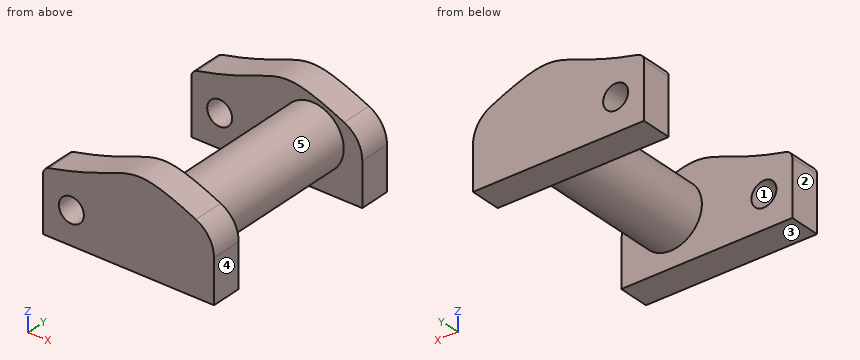
from build123d import *

# Parameters (mm, degrees)
F1_DEPTH = 25.4
F2_R     = 25.4
F3_DEPTH = 127
F6_R     = 25.3967781552
F7_R     = 10.211273354
F8_DEPTH = 211.42987


# Not quite as in the source:
# - a feature of the source that left no trace in its solid (it failed there, or was rolled back) is left out
# - a pattern or mirror of a feature is missing from the dataset's text; its kind, count and spacing are read off the source's solid


with BuildPart() as f1:
    # F0 (on Front) → F1 (new body)
    with BuildSketch(Plane.XZ):
        with BuildLine():
            Line((-140.086213054, 0), (0, 0))
            Line((0, 0), (0, 51.7864115536))
            add(Edge.make_bspline(
                [(-135.121182604, 51.4369904306), (-57.8541277154, 68.705081156), (-79.1493766813, 89.948796737), (0, 51.7864115536)],
                knots=[0.0132853618, 0.0132853618, 0.0132853618, 0.0132853618, 0.6502691411, 0.6502691411, 0.6502691411, 0.6502691411], degree=3))
            ThreePointArc((-135.121182604, 51.4369904306), (-138.6918692488, 49.210252186), (-140.086213054, 45.2398653435))
            Line((-140.086213054, 45.2398653435), (-140.086213054, 0))
        make_face()
    extrude(amount=F1_DEPTH)


with BuildPart() as f1_copies_1:
    # F1_copies: instance of F1
    add(f1.part.mirror(Plane(origin=(0, -88.9, 1e-06), x_dir=(0, 0, -1), z_dir=(0, -1, 0))))


with BuildPart() as f1_1:
    add(f1.part)

    add(f1_copies_1.part)  # F3 merges F1_copies_1
    # F2 (on face) → F3 (join)
    with BuildSketch(Plane.XZ.offset(25.4)):
        with Locations((-40.6125485897, 38.6877208911)):
            Circle(F2_R)
    extrude(amount=F3_DEPTH)

    # F6
    f6_edges = [f1_1.edges().sort_by_distance(p)[0] for p in [
        (0, -12.7, 51.786412),
        (0, -165.1, 51.786412),
    ]]
    fillet(f6_edges, radius=F6_R)

    # F7 (on face) → F8 (cut)
    with BuildSketch(Plane(origin=(0, 0, 0), x_dir=(-1, 0, 0), z_dir=(0, 1, 0))):
        with Locations((116.8357878923, 26.8229749054)):
            Circle(F7_R)
    extrude(amount=-F8_DEPTH, mode=Mode.SUBTRACT)


solid = f1_1.part
Source: CAD feature listing. Evaluate the final solid. Frame: model axes, mm. Face numbers are marked on the shaded views. A direction names the side the tool comes from. Coordinates: 2 decimals unless noted, no trailing zeros. Order: outer loops, then holes, each group sorted by start corner. A loop starts at its lowest first (then second) coordinate and runs counter-clockwise, first axis right, second up. Notation, with made-up numbers: M 68,86.5 L 117,86.5 A6 cw 117,95.5 Z; hole C -35,39 d2. An arc over 180 degrees is marked long. Write each question's results on one line, items separated by ' | '. Start each with the question number.
Item 1: Draft query along X for the marked faces 1, 2 and 3. Return one class per face: pulls with the +X half, pulls with the -X half, needs draft (parallel to the pull), parting line crosses it, or undercut.
Item 2: Line query: probe 1 along X at (y, z) = (-54.5, 38.5); probe 2 along X at (y, z) = (-159, 30); probe 3 along X at (y, z) = (-166, 31). Output: solid intervals per line, ascending.
Item 3: Set-up query: the marked faces 4 and 5. Return all of +Z, -Z, +X, -X, +Y, -Y with unobstructed straight access to the full face (end or side cutting, diameter ignored); none if empty.
Item 4: First-contact query: pin 1 Ø10 at (x, y) = (-40, -95) entering from -Z; pin 2 Ø10 at (y, z) = (-114, 44) entering from +X; pin 3 Ø8 at (y, z) = (-93.5, 29) entering from +X. Flat tips, straight axial feed; report the tip coordinate or a pass-through.
Item 5: Cut plane C-C (y = -32). Return loops of the section in (x, z).
Item 6: Cut plane A-A (z = 5). Return loops of the section in (x, y).
Item 7: Cut plane B-B (x = -124.5). Count the separate pieces of the cut face and the enclosed holes in it, and give its area (3 significant figures).
Checked values:
1) face 1: undercut | face 2: pulls with the -X half | face 3: needs draft
2) probe 1: x = -66.01 to -15.21 | probe 2: x = -140.09 to -126.54, -107.13 to 0 | probe 3: x = -140.09 to -126.15, -107.52 to 0
3) face 4: +Z, -Z, +X, +Y, -Y | face 5: none
4) pin 1: stops at z = 13.29 | pin 2: stops at x = -15.21 | pin 3: stops at x = -15.86
5) outline: C -40.61,38.69 d50.8
6) outline: M -140.09,-177.8 L 0,-177.8 L 0,-152.4 L -140.09,-152.4 Z; M -140.09,-25.4 L 0,-25.4 L 0,0 L -140.09,0 Z
7) separate pieces: 4 | enclosed holes: 0 | area: 2,060 mm2
